```python
from build123d import *

# Parameters (mm, degrees)
SKETCH1_R           = 7.8875
SKETCH1_R_2         = 2.5
SKETCH1_R_3         = 1.4
BOSS_EXTRUDE1_DEPTH = 4.5


with BuildPart() as part:
    # Sketch1 → Boss-Extrude1 (new body)
    with BuildSketch(Plane.XY):
        with BuildLine():
            Line((-9.955957701, -0.9375), (-17.422925977, 78.359375))
            ThreePointArc((-17.422925977, 78.359375), (0, 97.5), (17.422925977, 78.359375))
            Line((17.422925977, 78.359375), (9.955957701, -0.9375))
            ThreePointArc((9.955957701, -0.9375), (0, -10), (-9.955957701, -0.9375))
        make_face()
        with Locations((0, 80)):
            Circle(SKETCH1_R, mode=Mode.SUBTRACT)
        Circle(SKETCH1_R_2, mode=Mode.SUBTRACT)
        with Locations((0, 7)):
            Circle(SKETCH1_R_3, mode=Mode.SUBTRACT)
        with Locations((0, -7)):
            Circle(SKETCH1_R_3, mode=Mode.SUBTRACT)
    extrude(amount=BOSS_EXTRUDE1_DEPTH)


solid = part.part
```
For this review, take the finished solid that the model builds, in its own axes (mm). Give positions to 0.01 mm unless a question says otherwise; leave off trailing zeros. Loops run counter-clockwise (first coordinate to the right, second up) from the corner with the lowest first, then second, coordinate; pieces in that order, holes last. Notation, with made-up numbers: M 59,37 L 88,37 A27 ccw 88,54 Z; hole C 78.25,12.5 d10. An arc over 180 degrees is marked long. One line per item, written item: value. Start each with the question number.
Q1. Add section B-B (y = 80). Give the boundary of the cut face in (x, z).
Q2. Add section D-D (y = 7). Give the boundary of the cut face in (x, z).
Q3. For L1, parallel to Y at x = 0, z = 2.95; L2, parallel to Y at x = -1, z = 1.4; L3, parallel to X at y = 81.5, z = 1.4, list the stretches that pass through material, from the lowest coordinate up.
Q4. Add section A-A (x = 0). Give the boundary of the cut face in (y, z), and give its area (3 significant figures).
Q5. Draft analysis for pull direction Y (two halves, no side actions). For faces 1 (the face through (-1.71, 72.3, 2.22)), 2 (the face through (-0.303, 5.633, 2.218)), 3 (the face through (-13.637, 38.156, 2.218)), 4 (the face through (0, 45, 0)), state which applies: released by +Y, released by -Y, zero draft, split by the parting line, or undercut.
Q6. Add section C-C (z = 2.4). Give the boundary of the cut face in (x, y) (1 decimal), and give its area (3 significant figures).
Q7. Clearance check with flat-ended pins moving along their axes: pin 1 Ø4 at (x, y) = (0, 0) entering from -Z; pin 2 Ø1 at (x, y) = (-6, 38.5) entering from -Z. State where each tip first meets the part, or that it passes through.
Reply:
1. outline: M -17.5,0 L -7.89,0 L -7.89,4.5 L -17.5,4.5 Z; M 7.89,0 L 17.5,0 L 17.5,4.5 L 7.89,4.5 Z
2. outline: M -10.7,0 L -1.4,0 L -1.4,4.5 L -10.7,4.5 Z; M 1.4,0 L 10.7,0 L 10.7,4.5 L 1.4,4.5 Z
3. L1: -10 to -8.4, -5.6 to -2.5, 2.5 to 5.6, 8.4 to 72.11, 87.89 to 97.5
3. L2: -9.95 to -7.98, -6.02 to -2.29, 2.29 to 6.02, 7.98 to 72.18, 87.82 to 97.47
3. L3: -17.44 to -7.74, 7.74 to 17.44
4. outline: M -10,0 L -8.4,0 L -8.4,4.5 L -10,4.5 Z; M -5.6,0 L -2.5,0 L -2.5,4.5 L -5.6,4.5 Z; M 2.5,0 L 5.6,0 L 5.6,4.5 L 2.5,4.5 Z; M 8.4,0 L 72.11,0 L 72.11,4.5 L 8.4,4.5 Z; M 87.89,0 L 97.5,0 L 97.5,4.5 L 87.89,4.5 Z
4. area: 365 mm²
5. face 1: undercut
5. face 2: undercut
5. face 3: released by -Y
5. face 4: zero draft
6. outline: M -17.4,78.4 L -10,-0.9 A10 ccw 10,-0.9 L 17.4,78.4 A17.5 ccw long Z; hole C 0,80 d15.8; hole C 0,0 d5; hole C 0,-7 d2.8; hole C 0,7 d2.8
6. area: 2,620 mm²
7. pin 1: through
7. pin 2: z = 0
